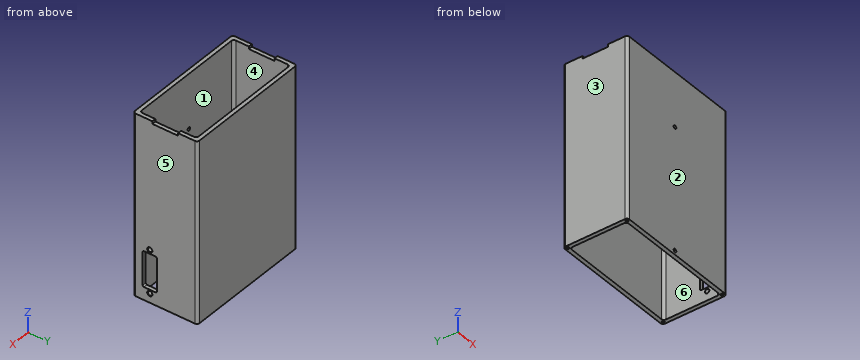
Autodesk Inventor part; units mm, degrees
ref_plane "YZ Plane" through (0, 0, 0) normal (1, 0, 0) x (0, 1, 0)
ref_plane "XZ Plane" through (0, 0, 0) normal (0, 1, 0) x (-1, 0, 0)
ref_plane "XY Plane" through (0, 0, 0) normal (0, 0, 1) x (1, 0, 0)
sketch "Sketch1" plane through (0, 0, 0) normal (0, 0, 1) x (1, 0, 0)
  line L0 (2, 0) -> (92, 0)
  line L1 (94, 2) -> (94, 42)
  line L2 (92, 44) -> (2, 44)
  line L3 (0, 42) -> (0, 2)
  line L4 (-1, 47) -> (95, 47)
  line L5 (97, 45) -> (97, -1)
  line L6 (95, -3) -> (-1, -3)
  line L7 (-3, -1) -> (-3, 45)
  arc A0 (2, 44) -> (0, 42) centre (2, 42) ccw
  arc A1 (0, 2) -> (2, 0) centre (2, 2) ccw
  arc A2 (92, 0) -> (94, 2) centre (92, 2) ccw
  arc A3 (94, 42) -> (92, 44) centre (92, 42) ccw
  arc A4 (-3, -1) -> (-1, -3) centre (-1, -1) ccw
  arc A5 (-1, 47) -> (-3, 45) centre (-1, 45) ccw
  arc A6 (97, 45) -> (95, 47) centre (95, 45) ccw
  arc A7 (95, -3) -> (97, -1) centre (95, -1) ccw
  point P0 (0, 0)
  point P1 (94, 44)
  point P2 (94, 0)
  point P3 (0, 44)
  point P4 (97, -3)
  point P5 (97, 47)
  point P6 (-3, -3)
  dimension "d0" = 94
  dimension "d1" = 44
  dimension "d2" = 100
  dimension "d3" = 50
  dimension "d4" = 3
  dimension "d5" = 3
  dimension "d6" = 2
  dimension "d9" = 2
extrude "Extrusion1" add sketch "Sketch1" along normal blind 140
sketch "Sketch2" plane through (0, 0, 140) normal (0, 0, 1) x (1, 0, 0)
  line L0 (-3, 45) -> (-3, -1)
  line L1 (97, -1) -> (97, 45)
  line L2 (-3, 32) -> (97, 32)
  line L3 (97, 32) -> (97, 12)
  line L4 (97, 12) -> (-3, 12)
  line L5 (-3, 12) -> (-3, 32)
  line L6 (-1, -3) -> (95, -3)
  line L7 (95, 47) -> (-1, 47)
  point P0 (0, 0)
  point P1 (-3, 12)
  dimension "d10" = 20
  dimension "d11" = 15
  dimension "d12" = 50
extrude "Extrusion2" cut sketch "Sketch2" against normal blind 2
sketch "Sketch3" plane through (97, -1, 0) normal (1, 0, 0) x (0, 0, -1)
  line L0 (-11, 5.5) -> (-36.5, 5.5)
  line L1 (-37.5, 6.5) -> (-37.5, 15.5)
  line L2 (-36.5, 16.5) -> (-11, 16.5)
  line L3 (-10, 15.5) -> (-10, 6.5)
  line L4 (0, -2) -> (-140, -2)
  line L5 (0, 48) -> (-140, 48)
  line L6 (0, 0) -> (0, 46)
  arc A0 (-11, 5.5) -> (-10, 6.5) centre (-11, 6.5) ccw
  arc A1 (-10, 15.5) -> (-11, 16.5) centre (-11, 15.5) ccw
  arc A2 (-37.5, 6.5) -> (-36.5, 5.5) centre (-36.5, 6.5) ccw
  arc A3 (-36.5, 16.5) -> (-37.5, 15.5) centre (-36.5, 15.5) ccw
  circle A4 centre (-7.09, 11) radius 1.5
  circle A5 centre (-40.41, 11) radius 1.5
  line L7 (-23.75, 5.5) -> (-23.75, 19.7829) construction
  point P0 (0, 1)
  point P1 (-37.5, 16.5)
  point P2 (-37.5, 5.5)
  point P3 (-10, 16.5)
  dimension "d15" = 27.5
  dimension "d16" = 11
  dimension "d17" = 50
  dimension "d18" = 31.5
  dimension "d19" = 10
  dimension "d20" = 1
  dimension "d21" = 3
  dimension "d22" = 3
  dimension "d23" = 16.66
  dimension "d24" = 16.66
extrude "Extrusion3" cut sketch "Sketch3" against normal blind 10 contours L0 A2 L1 A3 L2 A1 L3 A0
hole "Hole1" at (97, 10, 7.09) at (97, 10, 40.41) direction (-1, 0, 0) diameter 3.4 depth 8.8 tip angle 118
chamfer "Chamfer1" distance 0.3 angle 45 2 edges at (97, 10, 8.79) (97, 10, 42.11)
sketch "Sketch5" plane through (-1, -3, 0) normal (0, -1, 0) x (1, 0, 0)
  circle A0 centre (45.75, 3.13) radius 1.5
  circle A1 centre (45.75, 97.75) radius 1.5
  line L0 (98, 0) -> (98, 140)
  line L1 (0, 0) -> (96, 0)
  point P0 (1, 0)
  dimension "d49" = 3
  dimension "d50" = 3
  dimension "d51" = 94.62
  dimension "d52" = 52.25
  dimension "d53" = 3.13
hole "Hole3" at (44.75, -3, 3.13) at (44.75, -3, 97.75) direction (0, 1, 0) diameter 2.6416 depth 10.979 tip angle 118
sketch "Sketch6" plane through (0, 0, 0) normal (0, 0, -1) x (-1, 0, 0)
  circle A0 centre (0.8, -0.8) radius 1
  line L0 (1, -3) -> (-95, -3) construction
  line L1 (-47, -3) -> (-47, -11.0585) construction
  line L2 (3, 45) -> (3, -1) construction
  line L3 (3, 22) -> (17.9543, 22) construction
  circle A1 centre (0.8, 44.8) radius 1
  line L4 (-47, 47) -> (-47, 55.0585) construction
  circle A2 centre (-94.8, -0.8) radius 1
  circle A3 centre (-94.8, 44.8) radius 1
  point P0 (0, 0)
  point P1 (-94, 0)
  point P2 (-97, 45)
  point P3 (-97, -1)
  dimension "d61" = 2
  dimension "d62" = 2.2
  dimension "d63" = 2.2
hole "Hole4" at (-0.8, -0.8, 0) at (-0.8, 44.8, 0) at (94.8, 44.8, 0) at (94.8, -0.8, 0) direction (0, 0, 1) diameter 1.567 depth 4.5 tip angle 118
chamfer "Chamfer2" distance 0.2 angle 45 4 edges at (-0.8, -1.5835, 0) (-0.8, 44.0165, 0) (94.8, 44.0165, 0) (94.8, -1.5835, 0)
equation "\"d24\" = d23"
properties part number "obudowa"
Geometry check sheet. Reference: the model listing, model coordinates, mm. Face numbers are marked on the shaded views. A direction names the side the tool comes from. Round coordinates to 2 decimals unless told otherwise and drop trailing zeros. Write each loop counter-clockwise with the first axis right and the second up, starting at its lowest first coordinate (ties: lowest second). Pieces come first, ordered by that corner, then holes. Notation, with made-up numbers: (45, 55) -> (75, 55) arc R25 ccw to (75, 72) -> close; hole circle Ø10 at (87, -35.75). An arc over 180 degrees is marked (long way). Put each result on its own line as item: value.
1) Release check for a two-part mould opening along X. For the marked faces 1, 2, 3 and 4 record: pulls with the +X half, pulls with the -X half, needs draft (parallel to the pull), parting line crosses it, or undercut.
Recorded:
face 1: undercut
face 2: needs draft
face 3: pulls with the -X half
face 4: undercut
2) Thickness scan on probe 1 along Y at (x, z) = (94.8, 2.1); probe 2 along X at (y, z) = (44.8, 2); probe 3 along X at (y, z) = (37, 69). Record the ranges inside material, lowest first. Write a range as from..to.
Recorded:
probe 1: y = -3..-1.58, -0.02..44.02, 45.58..47
probe 2: x = -3..-1.58, -0.02..94.02, 95.58..97
probe 3: x = -3..0, 94..97
3) Access from +Z, -Z, +X, -X, +Y, -Y to the whole of each face (thin tool, end or side, straight path). Record for the marked faces 5 and 6.
Recorded:
face 5: +Z, -Z, +X, +Y, -Y
face 6: +Z, -Z
4) Cross-section at B-B, the plane x = 18. Enter the section's corners in (y, z), plus the area to 3 significant figures.
Recorded:
outline: (-3, 0) -> (0, 0) -> (0, 140) -> (-3, 140) -> close; (44, 0) -> (47, 0) -> (47, 140) -> (44, 140) -> close
area: 840 mm2
5) Depth check by flat-ended pin: P1, Ø1.6, axis at x = 44.75, z = 3.13, coming from the -Y side; P2, Ø0.9, axis at x = -0.8, y = 44.8, coming from the -Z side; P3, Ø1, axis at x = -2, z = 139.5, coming from the +Y side. Enter the tip coordinate at first touch or a pass-through.
Recorded:
P1: stops at y = 44
P2: stops at z = 4.7
P3: stops at y = 46.94
6) Cross-section at C-C, the plane z = 66.5. Enter the section's corners in (x, y), plus the area to 3 significant figures.
Recorded:
outline: (-3, -1) arc R2 ccw to (-1, -3) -> (95, -3) arc R2 ccw to (97, -1) -> (97, 45) arc R2 ccw to (95, 47) -> (-1, 47) arc R2 ccw to (-3, 45) -> close; hole (0, 2) arc R2 ccw to (2, 0) -> (92, 0) arc R2 ccw to (94, 2) -> (94, 42) arc R2 ccw to (92, 44) -> (2, 44) arc R2 ccw to (0, 42) -> close
area: 864 mm2
7) Cross-section at D-D, the plane z = 7.09. Enter the section's corners in (x, y), plus the area to 3 significant figures.
Recorded:
outline: (-3, -1) arc R2 ccw to (-1, -3) -> (95, -3) arc R2 ccw to (97, -1) -> (97, 8) -> (96.7, 8.3) -> (94, 8.3) -> (94, 2) arc R2 cw to (92, 0) -> (2, 0) arc R2 cw to (0, 2) -> (0, 42) arc R2 cw to (2, 44) -> (92, 44) arc R2 cw to (94, 42) -> (94, 11.7) -> (96.7, 11.7) -> (97, 12) -> (97, 45) arc R2 ccw to (95, 47) -> (-1, 47) arc R2 ccw to (-3, 45) -> close
area: 854 mm2
8) Cross-section at A-A, the plane y = 36. Enter the section's corners in (x, z), plus the area to 3 significant figures.
Recorded:
outline: (-3, 0) -> (0, 0) -> (0, 140) -> (-3, 140) -> close; (94, 0) -> (97, 0) -> (97, 140) -> (94, 140) -> close
area: 840 mm2
